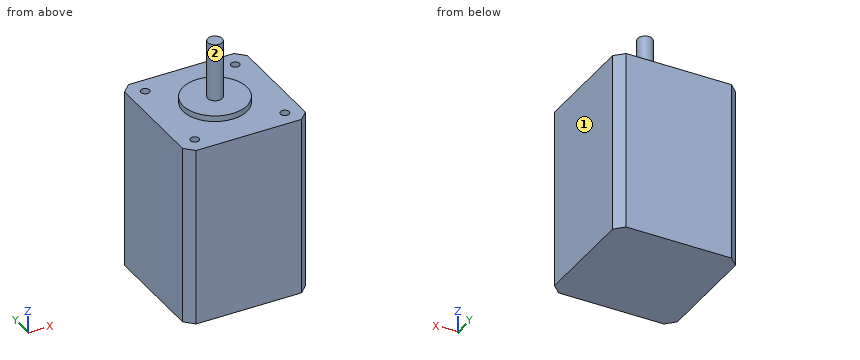
from build123d import *

# Parameters (mm, degrees)
SKETCH_1_W          = 42.3
SKETCH_1_H          = 42.3
EXTRUDE_1_DEPTH     = 62
SKETCH_2_R          = 11
EXTRUDE_2_DEPTH     = 2
SKETCH_3_R          = 2.5
EXTRUDE_3_DEPTH     = 20
CHAMFER_1_SIZE      = 3
SKETCH_4_R          = 1.5
CUT_EXTRUDE_1_DEPTH = 10


with BuildPart() as part:
    # 草图1 → 凸台-拉伸1 (new body)
    with BuildSketch(Plane.XY):
        Rectangle(SKETCH_1_W, SKETCH_1_H)
    extrude(amount=EXTRUDE_1_DEPTH)

    # 草图2 → 凸台-拉伸2 (add)
    with BuildSketch(Plane.XY.offset(62)):
        Circle(SKETCH_2_R)
    extrude(amount=EXTRUDE_2_DEPTH)

    # 草图3 → 凸台-拉伸3 (add)
    with BuildSketch(Plane.XY.offset(64)):
        Circle(SKETCH_3_R)
    extrude(amount=EXTRUDE_3_DEPTH)

    # 倒角1
    chamfer_1_edges = [part.edges().sort_by_distance(p)[0] for p in [
        (21.15, -21.15, 31),
        (-21.15, -21.15, 31),
        (-21.15, 21.15, 31),
        (21.15, 21.15, 31),
    ]]
    chamfer(chamfer_1_edges, length=CHAMFER_1_SIZE)

    # 草图4 → 切除-拉伸1 (cut)
    with BuildSketch(Plane.XY.offset(62)):
        with Locations((15.5, -15.5)):
            Circle(SKETCH_4_R)
        with Locations((-15.5, -15.5)):
            Circle(SKETCH_4_R)
        with Locations((15.5, 15.5)):
            Circle(SKETCH_4_R)
        with Locations((-15.5, 15.5)):
            Circle(SKETCH_4_R)
    extrude(amount=-CUT_EXTRUDE_1_DEPTH, mode=Mode.SUBTRACT)


solid = part.part
Can you work these out from the model? Positions are in its coordinate system, mm. Face numbers are marked on the shaded views. A direction names the side the tool comes from. Coordinates: 2 decimals unless noted, no trailing zeros. Order: outer loops, then holes, each group sorted by start corner. A loop starts at its lowest first (then second) coordinate and runs counter-clockwise, first axis right, second up. Notation, with made-up numbers: (-24.75, 75.25) - (-20.75, 75.25) arc R26 cw to (-20.75, 91.25) - close; hole circle Ø4 at (73.25, 12.25). An arc over 180 degrees is marked (long way). Answer as a JSON object with one key per item and string values. Group by question number.
Q1. I need wall thicknesses on line 1 (Y direction, x = -15.5, z = 59.75); line 2 (Y direction, x = -15, z = 55). Which ranges of each line are inside material? Lowest first, please. Write a range as from..to.
Q2. On a 3-axis mill with a long thin cutter (end or side, diameter ignored), from which of +Z, -Z, +X, -X, +Y, -Y can I reach the whole of each face in a straight line? I mean the marked faces 1 and 2. Say none if no direction works.
Q3. Imagine slicing it at D-D (z = 74). Please give me the cut outline in (x, y), and give its area (3 significant figures).
Q4. Imagine slicing it at A-A (z = 53). Please give me the cut outline in (x, y).
Q5. Will these pins go through, and if not, where does the flat tip stop? P1, Ø0.9, axis at x = -15, y = 15, coming from the +Z side; P2, Ø3.5, axis at x = 16, y = -15, coming from the +Z side.
Q6. Imagine slicing it at B-B (x = 0). Please give me the cut outline in (y, z).
Determined:
{
 "1": {"line 1": "y = -21.15..-17, -14..14, 17..21.15", "line 2": "y = -21.15..-16.91, -14.09..14.09, 16.91..21.15"},
 "2": {"face 1": "+Z, -Z, +X, +Y, -Y", "face 2": "+Z"},
 "3": {"outline": "circle Ø5 at (0, 0)", "area": "19.6 mm2"},
 "4": {"outline": "(-21.15, -18.15) - (-18.15, -21.15) - (18.15, -21.15) - (21.15, -18.15) - (21.15, 18.15) - (18.15, 21.15) - (-18.15, 21.15) - (-21.15, 18.15) - close; hole circle Ø3 at (-15.5, -15.5); hole circle Ø3 at (-15.5, 15.5); hole circle Ø3 at (15.5, -15.5); hole circle Ø3 at (15.5, 15.5)"},
 "5": {"P1": "stops at z = 52", "P2": "stops at z = 62"},
 "6": {"outline": "(-21.15, 0) - (21.15, 0) - (21.15, 62) - (11, 62) - (11, 64) - (2.5, 64) - (2.5, 84) - (-2.5, 84) - (-2.5, 64) - (-11, 64) - (-11, 62) - (-21.15, 62) - close"}
}
